```python
from build123d import *

# Parameters (mm, degrees)
F0_W      = 1120
F0_H      = 150
F1_DEPTH  = 50.8
F2_W      = 137.3
F2_H      = 88.9
F3_DEPTH  = 1120
F5_DEPTH  = 101.601
F7_DEPTH  = 101.601
F8_R      = 2.4
F9_W      = 101.6
F9_H      = 101.6
F10_DEPTH = 3.175
F11_R     = 2.5


with BuildPart() as f1:
    # F0 (on Top) → F1 (new body, symmetric)
    with BuildSketch(Plane.XY):
        Rectangle(F0_W, F0_H)
    extrude(amount=F1_DEPTH, both=True)

    # F2 (on face) → F3 (cut, through all)
    with BuildSketch(Plane(origin=(-560, 0, 0), x_dir=(0, -1, 0), z_dir=(-1, 0, 0))):
        Rectangle(F2_W, F2_H)
    extrude(amount=-F3_DEPTH, mode=Mode.SUBTRACT)

    # F4 (on face) → F5 (cut, through all)
    with BuildSketch(Plane.XY.offset(50.8)):
        Polygon((458.4, -75), (560, -75), (560, 75), align=None)
    extrude(amount=-F5_DEPTH, mode=Mode.SUBTRACT)

    # F6 (on face) → F7 (cut, through all)
    with BuildSketch(Plane.XY.offset(50.8)):
        Polygon((-560, 75), (-560, -75), (-458.4, -75), align=None)
    extrude(amount=-F7_DEPTH, mode=Mode.SUBTRACT)

    # F8
    f8_edges = [f1.edges().sort_by_distance(p)[0] for p in [
        (0, -75, 50.8),
        (0, -75, -50.8),
        (0, 75, -50.8),
        (0, 75, 50.8),
        (0, 68.65, -44.45),
        (0, 68.65, 44.45),
        (0, -68.65, 44.45),
        (0, -68.65, -44.45),
    ]]
    fillet(f8_edges, radius=F8_R)

    # F9 (on face) → F10 (cut)
    with BuildSketch(Plane.XY.offset(50.8)):
        with Locations((0, 0.8)):
            Rectangle(F9_W, F9_H)
    extrude(amount=-F10_DEPTH, mode=Mode.SUBTRACT)

    # F11
    f11_edges = [f1.edges().sort_by_distance(p)[0] for p in [
        (50.8, 51.6, 49.2125),
        (50.8, -50, 49.2125),
        (-50.8, -50, 49.2125),
        (-50.8, 51.6, 49.2125),
    ]]
    fillet(f11_edges, radius=F11_R)


solid = f1.part
```
Could you check a few things on this model? Use its own coordinates, in mm. A direction names the side the tool comes from. Coordinates: 2 decimals unless noted, no trailing zeros. Loops run counter-clockwise (first coordinate to the right, second up) from the corner with the lowest first, then second, coordinate; pieces in that order, holes last.
1) Imagine slicing it at B-B (x = 364). List the corners of the cut face in (y, z) for me.
Reported:
outline: (-75, -48.4) arc R2.4 ccw to (-72.6, -50.8) - (72.6, -50.8) arc R2.4 ccw to (75, -48.4) - (75, 48.4) arc R2.4 ccw to (72.6, 50.8) - (-72.6, 50.8) arc R2.4 ccw to (-75, 48.4) - close; hole (-68.65, -42.05) arc R2.4 ccw to (-66.25, -44.45) - (66.25, -44.45) arc R2.4 ccw to (68.65, -42.05) - (68.65, 42.05) arc R2.4 ccw to (66.25, 44.45) - (-66.25, 44.45) arc R2.4 ccw to (-68.65, 42.05) - close
2) Imagine slicing it at D-D (x = -480.5). List the corners of the cut face in (y, z) for me.
Reported:
outline: (-42.37, -50.8) - (72.6, -50.8) arc R2.4 ccw to (75, -48.4) - (75, 48.4) arc R2.4 ccw to (72.6, 50.8) - (-42.37, 50.8) - (-42.37, 44.45) - (66.25, 44.45) arc R2.4 cw to (68.65, 42.05) - (68.65, -42.05) arc R2.4 cw to (66.25, -44.45) - (-42.37, -44.45) - close
3) Imagine slicing it at C-C (y = -37). List the corners of the cut face in (x, z) for me (3 decimals), and give its area (3 significant figures).
Reported:
outline: (-484.139, -50.8) - (484.139, -50.8) - (484.139, -44.45) - (-484.139, -44.45) - close; (-484.139, 44.45) - (484.139, 44.45) - (484.139, 50.8) - (50.8, 50.8) - (50.8, 47.625) - (-50.8, 47.625) - (-50.8, 50.8) - (-484.139, 50.8) - close
area: 12,000 mm2
4) Which directions (+Z, -Z, +X, -X, +Y, -Y) give clear straight access to the entire face, cutting with the end or side of a thin tool? Please do faces 5 (the face through (-8, 68.65, -1)), 6 (the face through (-1, 2, 47.625)), 7 (the face through (-8, 75, 1)).
Reported:
face 5: +X, -X
face 6: +Z
face 7: +Z, -Z, +X, -X, +Y
5) Please list where these lines run through material, in increasing order: line 1 along Z through (x, y) = (-429.5, 37); line 2 along Y through (x, z) = (234, -30); line 3 along Y through (x, z) = (-459, 15.5).
Reported:
line 1: z = -50.8 to -44.45, 44.45 to 50.8
line 2: y = -75 to -68.65, 68.65 to 75
line 3: y = -74.11 to -68.65, 68.65 to 75
6) Will these pins go through, and if not, where does the flat tip stop? pin 1 Ø1 at (y, z) = (-22.5, 49.5) entering from +X; pin 2 Ø3.5 at (y, z) = (-15, 50) entering from -X; pin 3 Ø3.5 at (x, z) = (14.5, 49.5) entering from -Y; pin 4 Ø1 at (x, z) = (7, 49.5) entering from +Y.
Reported:
pin 1: stops at x = 494.3
pin 2: stops at x = -500.23
pin 3: stops at y = -75
pin 4: stops at y = 74.92
7) Thinking about a two-plate mould opening in Z: for faces 1 (the face through (-8, 66, 50.8)), 2 (the face through (-6, -75, 1)), 3 (the face through (-8, 1, -50.8)), 4 (the face through (-8, 1, 44.45)), which applies, released by +Z, released by -Z, zero draft, split by the parting line, or undercut?
Reported:
face 1: released by +Z
face 2: zero draft
face 3: released by -Z
face 4: undercut
8) Imagine slicing it at A-A (z = -31.5). List the corners of the cut face in (x, y) for me.
Reported:
outline: (-560, 75) - (-555.7, 68.65) - (555.7, 68.65) - (560, 75) - close; (-462.7, -68.65) - (-458.4, -75) - (458.4, -75) - (462.7, -68.65) - close
